Source: CAD feature listing. Evaluate the final solid. Frame: model axes, mm. Face numbers are marked on the shaded views. Give positions to 0.01 mm unless a question says otherwise; leave off trailing zeros. Loops run counter-clockwise (first coordinate to the right, second up) from the corner with the lowest first, then second, coordinate; pieces in that order, holes last. Notation, with made-up numbers: M 17,72.25 L 58,72.25 A17 ccw 58,103.25 Z; hole C -8,34.25 d7. An arc over 180 degrees is marked long. Answer in a Markdown table with one row per item.
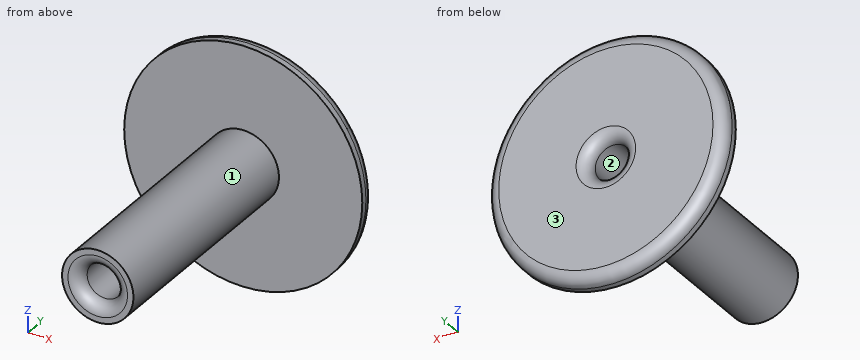
```python
from build123d import *

# Parameters (mm, degrees)
F2_R = 1


with BuildPart() as f1:
    # F0 (on Top) → F1 (revolve)
    with BuildSketch(Plane.XY):
        Polygon((-1.5, 0), (-10, 0), (-10, -1.5), (-3, -1.5), (-3, -21.5), (-1.5, -21.5), align=None)
    revolve(axis=Axis((0, -2.739727, 0), (0, -1, 0)))

    # F2
    f2_edges = [f1.edges().sort_by_distance(p)[0] for p in [
        (1.5, 0, 0),
        (10, 0, 0),
        (1.5, -21.5, 0),
    ]]
    fillet(f2_edges, radius=F2_R)


solid = f1.part
```
1) Section A-A, the plane z = 0. Return loops of the section in (x, y), then the cut area to 3 significant figures.
Reply:
| item | result |
|---|---|
| outline | M -10,-1.5 L -3,-1.5 L -3,-21.5 L -2.5,-21.5 A1 ccw -1.5,-20.5 L -1.5,-1 A1 ccw -2.5,0 L -9,0 A1 ccw -10,-1 Z; M 1.5,-20.5 A1 ccw 2.5,-21.5 L 3,-21.5 L 3,-1.5 L 10,-1.5 L 10,-1 A1 ccw 9,0 L 2.5,0 A1 ccw 1.5,-1 Z |
| area | 84.2 mm² |
2) Material intervals for L1, parallel to X at y = -13, z = 0; L2, parallel to Y at x = 6, z = -2.25, sorted ascending.
Reply:
| item | result |
|---|---|
| L1 | x = -3 to -1.5, 1.5 to 3 |
| L2 | y = -1.5 to 0 |
3) Section C-C, the plane y = -6. Return loops of the section in (x, z).
Reply:
| item | result |
|---|---|
| outline | C 0,0 d6; hole C 0,0 d3 |
4) Pull-direction query (Z, two-part tool) for the marked faces 1, 2 and 3; classes: released by +Z, released by -Z, zero draft, split by the parting line, or undercut.
Reply:
| item | result |
|---|---|
| face 1 | split by the parting line |
| face 2 | undercut |
| face 3 | zero draft |
5) Section B-B, the plane x = 0. Return loops of the section in (y, z).
Reply:
| item | result |
|---|---|
| outline | M -21.5,-3 L -1.5,-3 L -1.5,-10 L -1,-10 A1 ccw 0,-9 L 0,-2.5 A1 ccw -1,-1.5 L -20.5,-1.5 A1 ccw -21.5,-2.5 Z; M -21.5,2.5 A1 ccw -20.5,1.5 L -1,1.5 A1 ccw 0,2.5 L 0,9 A1 ccw -1,10 L -1.5,10 L -1.5,3 L -21.5,3 Z |
6) Pin query (flat end, axial travel): pin 1 Ø3.5 at (x, z) = (0, 0) entering from -Y; pin 2 Ø1 at (y, z) = (-3, 8) entering from -X; pin 3 Ø6 at (y, z) = (-10, -5) entering from -X; pin 4 Ø1.5 at (y, z) = (-2, 4.5) entering from +X. Return the tip coordinate at first contact, or that it passes through.
Reply:
| item | result |
|---|---|
| pin 1 | stops at y = -21.16 |
| pin 2 | passes through |
| pin 3 | stops at x = -2.24 |
| pin 4 | stops at x = 9.19 |
